Build history of the part. All positions in model axes, mm. Face numbers are marked on the shaded views. A direction names the side the tool comes from. Coordinates: 2 decimals unless noted, no trailing zeros. Order: outer loops, then holes, each group sorted by start corner. A loop starts at its lowest first (then second) coordinate and runs counter-clockwise, first axis right, second up. Notation, with made-up numbers: (73.25, 81.5) - (82.25, 81.5) arc R29 ccw to (82.25, 108.5) - close; hole circle Ø11 at (74, -21). An arc over 180 degrees is marked (long way). Return JSON: item names as keys, results as strings.
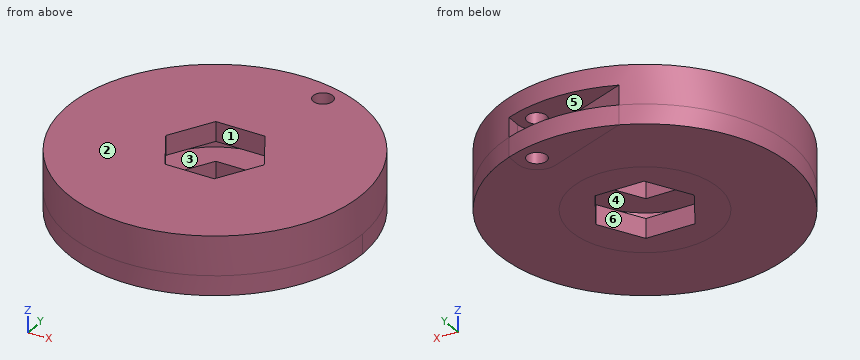
from build123d import *
from build123d.topology import SkipClean

# Parameters (mm, degrees)
SKETCH_1_R               = 15
EXTRUDE_1_DEPTH          = 6
CUT_EXTRUDE_1_DEPTH      = 23.045407685
SKETCH_5_R               = 7.5
CUT_EXTRUDE_2_DEPTH      = 23.045407685
EXTRUDE_START            = -2
SKETCH_6_R               = 15
EXTRUDE_4_DEPTH          = 2
SKETCH_7_R               = 15
EXTRUDE_5_DEPTH          = 2
CUT_EXTRUDE_3_DEPTH      = 22.587033145
CUT_EXTRUDE_3_DEPTH_BACK = 22.587033145
SKETCH_8_R               = 1
CUT_EXTRUDE_4_DEPTH      = 23.045407685


with BuildPart() as part:
    # Sketch 1 → Extrude 1 (new body)
    with BuildSketch(Plane.XY):
        Circle(SKETCH_1_R)
    extrude(amount=EXTRUDE_1_DEPTH)

    # Sketch 2 → Cut-Extrude 1 (cut, through all)
    with BuildSketch(Plane.XY.offset(6)):
        with BuildLine():
            Line((-5.64957048, 13.895407637), (2.749675697, 10.662349694))
            ThreePointArc((2.749675697, 10.662349694), (4.597345514, 10.878128051), (5.468121165, 12.521963144))
            Line((5.468121165, 12.521963144), (5.473092316, 13.965860536))
            ThreePointArc((5.473092316, 13.965860536), (-0.095010727, 14.999699096), (-5.64957048, 13.895407637))
        make_face()
    extrude(amount=-CUT_EXTRUDE_1_DEPTH, mode=Mode.SUBTRACT)

    # Sketch 5 → Cut-Extrude 2 (cut, through all)
    with BuildSketch(Plane.XY.offset(6)):
        Circle(SKETCH_5_R)
    extrude(amount=-CUT_EXTRUDE_2_DEPTH, mode=Mode.SUBTRACT)

    # Sketch 6 → Extrude 4 (add)
    with BuildSketch(Plane.XY.offset(6).offset(EXTRUDE_START)):
        with Locations(Location((0, 0, 0), (0, 0, 112.125589451))):
            Circle(SKETCH_6_R)
    extrude(amount=EXTRUDE_4_DEPTH)

    # Sketch 7 → Extrude 5 (add)
    with SkipClean():  # the faces are left unmerged after this step: merging them gives an invalid solid
        with BuildSketch(Plane(origin=(0, 0, 0), x_dir=(-1, 0, 0), z_dir=(0, 0, -1))):
            with Locations(Location((0, 0, 0), (0, 0, 180))):
                Circle(SKETCH_7_R)
        extrude(amount=-EXTRUDE_5_DEPTH)
    add(part.part.scale(1), mode=Mode.REPLACE)  # the faces are merged on a copy

    # Sketch 8 → Cut-Extrude 3 (cut, two sides: drawn at the far end of the back side and taken through both)
    with BuildSketch(Plane.XY.offset(2).offset(-CUT_EXTRUDE_3_DEPTH_BACK)):
        with Locations((3.468133018, 12.572519868)):
            Circle(SKETCH_8_R)
    extrude(amount=CUT_EXTRUDE_3_DEPTH + CUT_EXTRUDE_3_DEPTH_BACK, mode=Mode.SUBTRACT)

    # Sketch 9 → Cut-Extrude 4 (cut, through all)
    with BuildSketch(Plane.XY.offset(6)):
        Polygon((2.5, -4.330127019), (5, 0), (2.5, 4.330127019), (-2.5, 4.330127019), (-5, 0), (-2.5, -4.330127019), align=None)
    extrude(amount=-CUT_EXTRUDE_4_DEPTH, mode=Mode.SUBTRACT)


solid = part.part
1. Mould opens along Z. For the marked faces 1, 2 and 3 say: pulls with the +Z half, pulls with the -Z half, needs draft (parallel to the pull), parting line crosses it, or undercut.
Check values:
{"face 1": "needs draft", "face 2": "pulls with the +Z half", "face 3": "undercut"}
2. Cut at A-A on y = 2. Give the cut face in (x, z).
Check values:
{"outline": "(-14.87, 0) - (-3.85, 0) - (-3.85, 2) - (-7.23, 2) - (-7.23, 4) - (-3.85, 4) - (-3.85, 6) - (-14.87, 6) - close; (3.85, 0) - (14.87, 0) - (14.87, 6) - (3.85, 6) - (3.85, 4) - (7.23, 4) - (7.23, 2) - (3.85, 2) - close"}
3. Probe L1, parallel to Z at x = 4, y = -4.5; L2, parallel to X at y = -3.5, z = 2.25; L3, parallel to X at y = -1, z = 1.5. List the from-to ranges inside material, lowest first.
Check values:
{"L1": "0 to 2, 4 to 6", "L2": "-14.59 to -6.63, 6.63 to 14.59", "L3": "-14.97 to -4.42, 4.42 to 14.97"}
4. Cut at D-D on y = -3. Give the cut face in (x, z).
Check values:
{"outline": "(-14.7, 0) - (-3.27, 0) - (-3.27, 2) - (-6.87, 2) - (-6.87, 4) - (-3.27, 4) - (-3.27, 6) - (-14.7, 6) - close; (3.27, 0) - (14.7, 0) - (14.7, 6) - (3.27, 6) - (3.27, 4) - (6.87, 4) - (6.87, 2) - (3.27, 2) - close"}
5. Tool access for the marked faces 4, 5 and 6: list every direction of +Z, -Z, +X, -X, +Y, -Y with a clear straight run to the whole face (end or side of a thin tool).
Check values:
{"face 4": "none", "face 5": "+Y", "face 6": "+Z, -Z"}
6. Cut at B-B on z = 3.5. Give the cut face in (x, y), plus the area to 3 significant figures.
Check values:
{"outline": "(-5.65, 13.9) arc R15 ccw (long way) to (5.47, 13.97) - (5.47, 12.52) arc R2 cw to (2.75, 10.66) - close; hole circle Ø15 at (0, 0)", "area": "500 mm²"}
7. Drop flat-ended pins along their axis: pin 1 (3 mm diameter, centred on y = -4.5, z = 1.5, fed in from -X); pin 2 (3 mm diameter, centred on x = 11.5, z = 1.5, fed in from +Y); pin 3 (1.6 mm diameter, centred on x = 1, z = 5, fed in from -Y). Give the stop position or say it passes through.
Check values:
{"pin 1": "x = -14.7", "pin 2": "y = 11.18", "pin 3": "y = -15"}
8. Cut at C-C on x = 0. Give the cut face in (y, z).
Check values:
{"outline": "(-15, 0) - (-4.33, 0) - (-4.33, 2) - (-7.5, 2) - (-7.5, 4) - (-4.33, 4) - (-4.33, 6) - (-15, 6) - close; (4.33, 0) - (15, 0) - (15, 2) - (11.72, 2) - (11.72, 4) - (15, 4) - (15, 6) - (4.33, 6) - (4.33, 4) - (7.5, 4) - (7.5, 2) - (4.33, 2) - close"}
